```python
from build123d import *

# Parameters (mm, degrees)
BOSS_EXTRUDE1_START     = 2
SKETCH1_W               = 175
SKETCH1_H               = 126
BOSS_EXTRUDE1_DEPTH     = 2
SKETCH2_R               = 5
BOSS_EXTRUDE2_DEPTH     = 2
FILLET1_R               = 2
BOSS_EXTRUDE3_DEPTH     = 15.65
CUT_EXTRUDE_THIN1_DEPTH = 2.25
SKETCH8_R               = 4
BOSS_EXTRUDE4_DEPTH     = 17.65
FILLET2_R               = 8


with BuildPart() as part:
    # Sketch1 → Boss-Extrude1 (new body)
    with BuildSketch(Plane.XY.offset(BOSS_EXTRUDE1_START)):
        with Locations((-70.5, 46)):
            Rectangle(SKETCH1_W, SKETCH1_H)
    extrude(amount=BOSS_EXTRUDE1_DEPTH)

    # Sketch2 → Boss-Extrude2 (add)
    with BuildSketch(Plane(origin=(0, 0, 2), x_dir=(-1, 0, 0), z_dir=(0, 0, -1))):
        Circle(SKETCH2_R)
        with Locations((69.5, 63.5)):
            Circle(SKETCH2_R)
        with Locations((0, 92)):
            Circle(SKETCH2_R)
        with Locations((141, 92)):
            Circle(SKETCH2_R)
        with Locations((141, 0)):
            Circle(SKETCH2_R)
    extrude(amount=BOSS_EXTRUDE2_DEPTH)

    # Fillet1
    fillet1_edges = [part.edges().sort_by_distance(p)[0] for p in [
        (-158, 109, 3),
        (17, 109, 3),
        (17, -17, 3),
        (-158, -17, 3),
    ]]
    fillet(fillet1_edges, radius=FILLET1_R)

    # Sketch3 → Boss-Extrude3 (add)
    with BuildSketch(Plane(origin=(0, 0, 2), x_dir=(-1, 0, 0), z_dir=(0, 0, -1))):
        with BuildLine():
            Line((-15, 109), (156, 109))
            ThreePointArc((156, 109), (157.414213562, 108.414213562), (158, 107))
            Line((158, 107), (158, -15))
            ThreePointArc((158, -15), (157.414213562, -16.414213562), (156, -17))
            Line((156, -17), (-15, -17))
            ThreePointArc((-15, -17), (-16.414213562, -16.414213562), (-17, -15))
            Line((-17, -15), (-17, 107))
            ThreePointArc((-17, 107), (-16.414213562, 108.414213562), (-15, 109))
        make_face()
        with BuildLine():
            Line((-3, 102), (144, 102))
            ThreePointArc((144, 102), (148.949747468, 99.949747468), (151, 95))
            Line((151, 95), (151, -3))
            ThreePointArc((151, -3), (148.949747468, -7.949747468), (144, -10))
            Line((144, -10), (-3, -10))
            ThreePointArc((-3, -10), (-7.949747468, -7.949747468), (-10, -3))
            Line((-10, -3), (-10, 95))
            ThreePointArc((-10, 95), (-7.949747468, 99.949747468), (-3, 102))
        make_face(mode=Mode.SUBTRACT)
    extrude(amount=BOSS_EXTRUDE3_DEPTH)

    # Sketch5 → Cut-Extrude-Thin1 (cut)
    with BuildSketch(Plane(origin=(0, 0, -13.65), x_dir=(-1, 0, 0), z_dir=(0, 0, -1))):
        with BuildLine():
            Line((-3, 107), (144, 107))
            ThreePointArc((144, 107), (152.485281374, 103.485281374), (156, 95))
            Line((156, 95), (156, -3))
            ThreePointArc((156, -3), (152.485281374, -11.485281374), (144, -15))
            Line((144, -15), (-3, -15))
            ThreePointArc((-3, -15), (-11.485281374, -11.485281374), (-15, -3))
            Line((-15, -3), (-15, 95))
            ThreePointArc((-15, 95), (-11.485281374, 103.485281374), (-3, 107))
        make_face()
        with BuildLine():
            Line((-3, 104), (144, 104))
            ThreePointArc((144, 104), (150.363961031, 101.363961031), (153, 95))
            Line((153, 95), (153, -3))
            ThreePointArc((153, -3), (150.363961031, -9.363961031), (144, -12))
            Line((144, -12), (-3, -12))
            ThreePointArc((-3, -12), (-9.363961031, -9.363961031), (-12, -3))
            Line((-12, -3), (-12, 95))
            ThreePointArc((-12, 95), (-9.363961031, 101.363961031), (-3, 104))
        make_face(mode=Mode.SUBTRACT)
    extrude(amount=-CUT_EXTRUDE_THIN1_DEPTH, mode=Mode.SUBTRACT)

    # Sketch8 → Boss-Extrude4 (add)
    with BuildSketch(Plane(origin=(0, 0, -13.65), x_dir=(-1, 0, 0), z_dir=(0, 0, -1))):
        with Locations((156, 107)):
            Circle(SKETCH8_R)
        with Locations((156, -15)):
            Circle(SKETCH8_R)
        with Locations((-15, -15)):
            Circle(SKETCH8_R)
        with Locations((-15, 107)):
            Circle(SKETCH8_R)
    extrude(amount=-BOSS_EXTRUDE4_DEPTH)

    # Fillet2
    fillet2_edges = [part.edges().sort_by_distance(p)[0] for p in [
        (-152.535898385, 109, -4.825),
        (-158, 103.535898385, -4.825),
        (-158, -11.535898385, -4.825),
        (-152.535898385, -17, -4.825),
        (11.535898385, -17, -4.825),
        (17, -11.535898385, -4.825),
        (11.535898385, 109, -4.825),
        (17, 103.535898385, -4.825),
    ]]
    fillet(fillet2_edges, radius=FILLET2_R)


solid = part.part
```
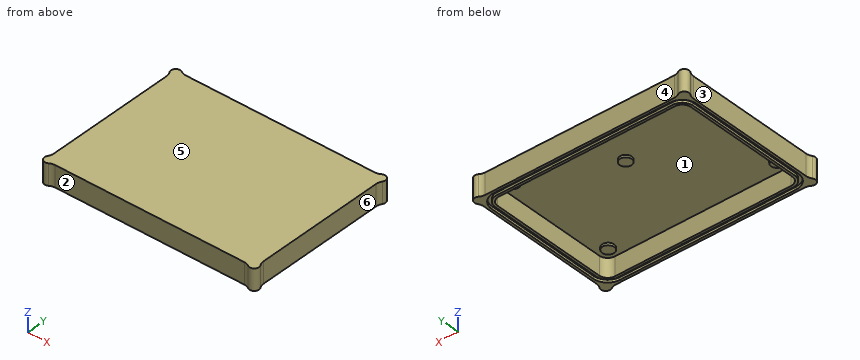
Verification items for the finished model (mm, model axes). Face numbers are marked on the shaded views. A direction names the side the tool comes from. Coordinates: 2 decimals unless noted, no trailing zeros. Loops run counter-clockwise (first coordinate to the right, second up) from the corner with the lowest first, then second, coordinate; pieces in that order, holes last. Notation, with made-up numbers: (63, 6.25) -> (115, 6.25) arc R21 cw to (115, 38.25) -> close; hole circle Ø4 at (21.25, 75.25). An arc over 180 degrees is marked (long way). Answer in a Markdown table with one row per item. Add a question column.
1. Section check C-C, the plane y = 92. Enter the section's corners in (x, z).
2. Section check D-D, the plane x = -141. Enter the section's corners in (y, z).
3. Depth check by flat-ended pin: P1, Ø5.5, axis at y = 69, z = -5.5, coming from the +X side; P2, Ø11, axis at x = -141, y = -0.5, coming from the -Z side; P3, Ø2.5, axis at y = 62, z = -12.5, coming from the -X side. Enter the tip coordinate at first touch or a pass-through.
4. Material ranges on probe 1 along Y at (x, z) = (-14, -12); probe 2 along X at (y, z) = (49, -6); probe 3 along X at (y, z) = (4, -11.75), recorded low to high. Write a range as [from, to].
5. Section check A-A, the plane z = -5.75. Enter the section's corners in (x, y), then the cut area to 3 significant figures.
6. Access from +Z, -Z, +X, -X, +Y, -Y to the whole of each face (thin tool, end or side, straight path). Record for the marked faces 1, 2 and 3.
7. Draft check along Y on the marked faces 4, 5 and 6. Enter one of: +Y half, -Y half, draft (parallel to the pull), parting line (faces both ways), or undercut.
8. Section check B-B, the plane x = -122. Enter the section's corners in (y, z).
Derived:
| question | item | result |
|---|---|---|
| 1 | outline | (-158, -13.65) -> (-156, -13.65) -> (-156, -11.4) -> (-153, -11.4) -> (-153, -13.65) -> (-151, -13.65) -> (-151, 2) -> (-146, 2) -> (-146, 0) -> (-136, 0) -> (-136, 2) -> (-5, 2) -> (-5, 0) -> (5, 0) -> (5, 2) -> (10, 2) -> (10, -13.65) -> (12, -13.65) -> (12, -11.4) -> (15, -11.4) -> (15, -13.65) -> (17, -13.65) -> (17, 4) -> (-158, 4) -> close |
| 2 | outline | (-17, -13.65) -> (-15, -13.65) -> (-15, -11.4) -> (-12, -11.4) -> (-12, -13.65) -> (-10, -13.65) -> (-10, 2) -> (-5, 2) -> (-5, 0) -> (5, 0) -> (5, 2) -> (87, 2) -> (87, 0) -> (97, 0) -> (97, 2) -> (102, 2) -> (102, -13.65) -> (104, -13.65) -> (104, -11.4) -> (107, -11.4) -> (107, -13.65) -> (109, -13.65) -> (109, 4) -> (-17, 4) -> close |
| 3 | P1 | stops at x = 17 |
| 3 | P2 | stops at z = 0 |
| 3 | P3 | stops at x = -158 |
| 4 | probe 1 | y = [-17, -15], [-12, -10], [102, 104], [107, 109] |
| 4 | probe 2 | x = [-158, -151], [10, 17] |
| 4 | probe 3 | x = [-158, -156], [-153, -151], [10, 12], [15, 17] |
| 5 | outline | (-159.33, -12.79) arc R4 ccw to (-153.79, -18.33) arc R8 cw to (-149.37, -17) -> (8.37, -17) arc R8 cw to (12.79, -18.33) arc R4 ccw to (18.33, -12.79) arc R8 cw to (17, -8.37) -> (17, 100.37) arc R8 cw to (18.33, 104.79) arc R4 ccw to (12.79, 110.33) arc R8 cw to (8.37, 109) -> (-149.37, 109) arc R8 cw to (-153.79, 110.33) arc R4 ccw to (-159.33, 104.79) arc R8 cw to (-158, 100.37) -> (-158, -8.37) arc R8 cw to start; hole (-151, -3) arc R7 ccw to (-144, -10) -> (3, -10) arc R7 ccw to (10, -3) -> (10, 95) arc R7 ccw to (3, 102) -> (-144, 102) arc R7 ccw to (-151, 95) -> close |
| 5 | area | 4,140 mm² |
| 6 | face 1 | -Z |
| 6 | face 2 | +Z, -Z, -Y |
| 6 | face 3 | +Z, -Z, -X |
| 7 | face 4 | +Y half |
| 7 | face 5 | draft |
| 7 | face 6 | undercut |
| 8 | outline | (-17, -13.65) -> (-15, -13.65) -> (-15, -11.4) -> (-12, -11.4) -> (-12, -13.65) -> (-10, -13.65) -> (-10, 2) -> (102, 2) -> (102, -13.65) -> (104, -13.65) -> (104, -11.4) -> (107, -11.4) -> (107, -13.65) -> (109, -13.65) -> (109, 4) -> (-17, 4) -> close |
